For this review, take the finished solid that the model builds, in its own axes (mm). A direction names the side the tool comes from. Give positions to 0.01 mm unless a question says otherwise; leave off trailing zeros. Loops run counter-clockwise (first coordinate to the right, second up) from the corner with the lowest first, then second, coordinate; pieces in that order, holes last. Notation, with made-up numbers: (-31.75, -0.75) -> (9.25, -0.75) arc R25 ccw to (9.25, 27.25) -> close; hole circle Ø5 at (13.5, 17.25). An arc over 180 degrees is marked (long way). One line per question, with ' | ' between items. Start each with the question number.
(1) Draft analysis for pull direction Y (two halves, no side actions). For faces 3 (the flat face through (-4.1, 3.2, 10)), 4 (the cylindrical face through (-8, -6, 5)), state which applies: +Y half, -Y half, draft (parallel to the pull), parting line (faces both ways), or undercut.
(2) Tool access review of faces 1 (the cylindrical face through (10, 0, 5)), 2 (the cylindrical face through (8, -6, 5)): name each direction out of +Z, -Z, +X, -X, +Y, -Y from which nothing blocks a thin tool from reaching the whole face with its end or side.
(3) Insertion check: P1, Ø5, axis at x = 8.5, y = 9, coming from the -Z side; P2, Ø1, axis at x = -4, y = -8.5, coming from the +Z side; P3, Ø1, axis at x = -8, z = 5, coming from the -Y side. Each pin has a flat end and moves straight along its axis. Give the tip position at first contact, or say it passes through.
(4) Wall thickness on probe 1 along Y at (x, z) = (0, 3); probe 2 along X at (y, z) = (10, 4); probe 3 along X at (y, z) = (0, 7): over which ranges is each line inside the solid? List them lowest first.
(5) Consider section C-C (z = 1.75). Write out the cut boundary in (x, y).
(6) Consider section D-D (x = -8). Write out the cut boundary in (y, z), and give its area (3 significant figures).
(7) Consider section B-B (x = 0). Write out the cut boundary in (y, z), and give its area (3 significant figures).
(8) Consider section A-A (y = 0). Write out the cut boundary in (x, z).
from build123d import *

# Parameters (mm, degrees)
SKIZZE1_R                            = 10
AUFSATZ_LINEAR_AUSTRAGEN1_DEPTH      = 10
AUFSATZ_LINEAR_AUSTRAGEN4_DEPTH      = 0.5
AUFSATZ_LINEAR_AUSTRAGEN4_DEPTH_BACK = 10.5
SKIZZE5_R                            = 5
SKIZZE2_R                            = 2.5
AUFSATZ_LINEAR_AUSTRAGEN2_DEPTH      = 10
KREISMUSTER1_COUNT                   = 10
SCHNITT_LINEAR_AUSTRAGEN1_DEPTH      = 0.5
SCHNITT_LINEAR_AUSTRAGEN1_DEPTH_BACK = 20
SKIZZE3_R                            = 2.5
SKIZZE4_W                            = 3.121683878
SKIZZE4_H                            = 1.135727963
AUFSATZ_LINEAR_AUSTRAGEN3_DEPTH      = 10


with BuildPart() as part:
    # Skizze1 → Aufsatz-Linear austragen1 (new body)
    with BuildSketch(Plane.XY):
        Circle(SKIZZE1_R)
    extrude(amount=AUFSATZ_LINEAR_AUSTRAGEN1_DEPTH)

    # Skizze5 → Aufsatz-Linear austragen4 (add, two sides: drawn at the far end of the back side and taken through both)
    with BuildSketch(Plane.XY.offset(10).offset(-AUFSATZ_LINEAR_AUSTRAGEN4_DEPTH_BACK)):
        Circle(SKIZZE5_R)
    extrude(amount=AUFSATZ_LINEAR_AUSTRAGEN4_DEPTH + AUFSATZ_LINEAR_AUSTRAGEN4_DEPTH_BACK)

    # Skizze2 → Aufsatz-Linear austragen2 (add)
    with BuildSketch(Plane(origin=(0, 0, 0), x_dir=(-1, 0, 0), z_dir=(0, 0, -1))):
        with Locations((0, 10)):
            Circle(SKIZZE2_R)
    aufsatz_linear_austragen2 = extrude(amount=-AUFSATZ_LINEAR_AUSTRAGEN2_DEPTH)

    # Kreismuster1: Aufsatz-Linear austragen2 ×10 about axis
    kreismuster1_axis = Axis((0, 0, 0), (0, 0, 1))
    for i in range(1, KREISMUSTER1_COUNT):
        add(aufsatz_linear_austragen2.rotate(kreismuster1_axis, i * 360 / KREISMUSTER1_COUNT))

    # Skizze3 → Schnitt-Linear austragen1 (cut, two sides: drawn at the far end of the back side and taken through both)
    with BuildSketch(Plane.XY.offset(10).offset(-SCHNITT_LINEAR_AUSTRAGEN1_DEPTH_BACK)):
        Circle(SKIZZE3_R)
    extrude(amount=SCHNITT_LINEAR_AUSTRAGEN1_DEPTH + SCHNITT_LINEAR_AUSTRAGEN1_DEPTH_BACK, mode=Mode.SUBTRACT)

    # Skizze4 → Aufsatz-Linear austragen3 (add)
    with BuildSketch(Plane.XY.offset(10)):
        with Locations((0.060841939, -2.567863982)):
            Rectangle(SKIZZE4_W, SKIZZE4_H)
    extrude(amount=-AUFSATZ_LINEAR_AUSTRAGEN3_DEPTH)


solid = part.part
A:
1) face 3: draft | face 4: undercut
2) face 1: +Z, -Z, +X | face 2: +Z, -Z
3) P1: stops at z = 0 | P2: stops at z = 10 | P3: stops at y = -9.99
4) probe 1: y = -12.5 to -2, 2.5 to 12.5 | probe 2: x = -7.49 to -4.26, -2.5 to 2.5, 4.26 to 7.49 | probe 3: x = -10 to -2.5, 2.5 to 10
5) outline: (-9.98, -0.63) arc R2.5 ccw (long way) to (-8.45, -5.35) arc R10 ccw to (-7.7, -6.38) arc R2.5 ccw (long way) to (-3.69, -9.3) arc R10 ccw to (-2.48, -9.69) arc R2.5 ccw (long way) to (2.48, -9.69) arc R10 ccw to (3.69, -9.3) arc R2.5 ccw (long way) to (7.7, -6.38) arc R10 ccw to (8.45, -5.35) arc R2.5 ccw (long way) to (9.98, -0.63) arc R10 ccw to (9.98, 0.63) arc R2.5 ccw (long way) to (8.45, 5.35) arc R10 ccw to (7.7, 6.38) arc R2.5 ccw (long way) to (3.69, 9.3) arc R10 ccw to (2.48, 9.69) arc R2.5 ccw (long way) to (-2.48, 9.69) arc R10 ccw to (-3.69, 9.3) arc R2.5 ccw (long way) to (-7.7, 6.38) arc R10 ccw to (-8.45, 5.35) arc R2.5 ccw (long way) to (-9.98, 0.63) arc R10 ccw to start; hole (-1.5, -2) -> (1.5, -2) arc R2.5 ccw (long way) to start
6) outline: (-9.41, 0) -> (-6.77, 0) -> (-6.77, 10) -> (-9.41, 10) -> close; (-6, 0) -> (6, 0) -> (6, 10) -> (-6, 10) -> close; (6.77, 0) -> (9.41, 0) -> (9.41, 10) -> (6.77, 10) -> close | area: 173 mm^2
7) outline: (-12.5, 0) -> (-5, 0) -> (-5, -0.5) -> (-2.5, -0.5) -> (-2.5, 0) -> (-2, 0) -> (-2, 10) -> (-2.5, 10) -> (-2.5, 10.5) -> (-5, 10.5) -> (-5, 10) -> (-12.5, 10) -> close; (2.5, -0.5) -> (5, -0.5) -> (5, 0) -> (12.5, 0) -> (12.5, 10) -> (5, 10) -> (5, 10.5) -> (2.5, 10.5) -> close | area: 210 mm^2
8) outline: (-10, 0) -> (-5, 0) -> (-5, -0.5) -> (-2.5, -0.5) -> (-2.5, 10.5) -> (-5, 10.5) -> (-5, 10) -> (-10, 10) -> close; (2.5, -0.5) -> (5, -0.5) -> (5, 0) -> (10, 0) -> (10, 10) -> (5, 10) -> (5, 10.5) -> (2.5, 10.5) -> close
